```python
from build123d import *

# Parameters (mm, degrees)
SKETCH092_W             = 30.8
SKETCH092_H             = 12.5
PAD112_DEPTH            = 0.3
POCKET002_DEPTH         = 0.3
PAD113_DEPTH            = 5.5
POCKET003_DEPTH         = 5.5
FILLET014_R             = 0.75
SKETCH011_R             = 1.5
PAD114_DEPTH            = 5
BODY029_PLACEMENT_ANGLE = 180


with BuildPart() as part:
    # Sketch092 → Pad112 (new body)
    with BuildSketch(Plane(origin=(0, 3, 0), x_dir=(-1, 0, 0), z_dir=(0, 1, 0))):
        with Locations((0, 6.25)):
            Rectangle(SKETCH092_W, SKETCH092_H)
    extrude(amount=PAD112_DEPTH)

    # Sketch091 → Pocket002 (cut)
    with BuildSketch(Plane(origin=(0, 3, 0), x_dir=(-1, 0, 0), z_dir=(0, 1, 0))):
        with BuildLine():
            Line((-7, 10.175), (7, 10.175))
            ThreePointArc((7.391964, 9.675), (7.317662, 10.020388), (7, 10.175))
            Line((7.391964, 9.675), (5.67688, 2.69884))
            ThreePointArc((5.2, 2.325), (5.502973, 2.4296), (5.67688, 2.69884))
            Line((5.2, 2.325), (-5.2, 2.325))
            ThreePointArc((-5.67688, 2.69884), (-5.502973, 2.4296), (-5.2, 2.325))
            Line((-5.67688, 2.69884), (-7.391964, 9.675))
            ThreePointArc((-7, 10.175), (-7.317662, 10.020388), (-7.391964, 9.675))
        make_face()
    extrude(amount=POCKET002_DEPTH, mode=Mode.SUBTRACT)

    # Sketch091 → Pad113 (join)
    with BuildSketch(Plane(origin=(0, 3, 0), x_dir=(-1, 0, 0), z_dir=(0, 1, 0))):
        with BuildLine():
            Line((-7, 10.175), (7, 10.175))
            ThreePointArc((7.391964, 9.675), (7.317662, 10.020388), (7, 10.175))
            Line((7.391964, 9.675), (5.67688, 2.69884))
            ThreePointArc((5.2, 2.325), (5.502973, 2.4296), (5.67688, 2.69884))
            Line((5.2, 2.325), (-5.2, 2.325))
            ThreePointArc((-5.67688, 2.69884), (-5.502973, 2.4296), (-5.2, 2.325))
            Line((-5.67688, 2.69884), (-7.391964, 9.675))
            ThreePointArc((-7, 10.175), (-7.317662, 10.020388), (-7.391964, 9.675))
        make_face()
    extrude(amount=PAD113_DEPTH)

    # Sketch093 → Pocket003 (cut)
    with BuildSketch(Plane(origin=(0, 3, 0), x_dir=(-1, 0, 0), z_dir=(0, 1, 0))):
        with BuildLine():
            Line((-6, 9.18), (6, 9.18))
            ThreePointArc((6.390856, 8.68), (6.31732, 9.025285), (6, 9.18))
            Line((6.390856, 8.68), (5.098578, 3.485231))
            ThreePointArc((4.9, 3.33), (5.026026, 3.373413), (5.098578, 3.485231))
            Line((4.9, 3.33), (-4.9, 3.33))
            ThreePointArc((-5.098578, 3.485231), (-5.026026, 3.373413), (-4.9, 3.33))
            Line((-5.098578, 3.485231), (-6.390856, 8.68))
            ThreePointArc((-6, 9.18), (-6.31732, 9.025285), (-6.390856, 8.68))
        make_face()
    extrude(amount=POCKET003_DEPTH, mode=Mode.SUBTRACT)

    # Fillet014
    fillet014_edges = [part.edges().sort_by_distance(p)[0] for p in [
        (0, 8.5, 10.175),
        (7.317662, 8.5, 10.020388),
        (6.534422, 8.5, 6.18692),
        (5.502973, 8.5, 2.4296),
        (0, 8.5, 2.325),
        (-5.502973, 8.5, 2.4296),
        (-6.534422, 8.5, 6.18692),
        (-7.317662, 8.5, 10.020388),
    ]]
    fillet(fillet014_edges, radius=FILLET014_R)

    # Sketch011 → Pad114 (join)
    with BuildSketch(Plane(origin=(0, 3.3, 0), x_dir=(-1, 0, 0), z_dir=(0, 1, 0))):
        Polygon((-9.9, 4.893227), (-9.9, 7.606773), (-12.25, 8.963546), (-14.6, 7.606773), (-14.6, 4.893227), (-12.25, 3.536454), align=None)
        with Locations((-12.25, 6.25)):
            Circle(SKETCH011_R, mode=Mode.SUBTRACT)
        Polygon((14.6, 4.893227), (14.6, 7.606773), (12.25, 8.963546), (9.9, 7.606773), (9.9, 4.893227), (12.25, 3.536454), align=None)
        with Locations((12.25, 6.25)):
            Circle(SKETCH011_R, mode=Mode.SUBTRACT)
    extrude(amount=PAD114_DEPTH)


with BuildPart() as part_1:
    # Body029 placement: moved
    add(part.part.moved(Location((5.3, 0, 0))).rotate(Axis((5.3, 0, 0), (0, 0, 1)), BODY029_PLACEMENT_ANGLE))


solid = part_1.part
```
CAD build for the part. Positions are in the model's coordinates, mm. A direction names the side the tool comes from. Coordinates: 2 decimals unless noted, no trailing zeros. Order: outer loops, then holes, each group sorted by start corner. A loop starts at its lowest first (then second) coordinate and runs counter-clockwise, first axis right, second up. Notation, with made-up numbers: (-31.75, 35.25) - (18.25, 35.25) arc R22 cw to (18.25, 68.25) - close; hole circle Ø9 at (-33, 41). An arc over 180 degrees is marked (long way). Answer in a Markdown table with one row per item.
1. Pull direction Z, two halves, no side cores. Call faces 5 (the face through (11.054, -5.712, 6.119)), 6 (the face through (5, -5, 2.325)), 7 (the face through (16.4, -5.8, 8.3)): +Z half, -Z half, draft (parallel to the pull), parting line (faces both ways), or undercut.
Answer:
| item | result |
|---|---|
| face 5 | undercut |
| face 6 | -Z half |
| face 7 | +Z half |
2. 3-axis set-ups, long thin cutter, end or side, ignore diameter. For faces 1 (the face through (-8.1, -5.8, 8.3)), 2 (the face through (19.9, -6, 6)), 3 (the face through (-0.436, -5.712, 6.046)), 4 (the face through (18, -3.3, 6)): which of +Z, -Z, +X, -X, +Y, -Y reach the whole face in a straight line?
Answer:
| item | result |
|---|---|
| face 1 | +Z, -X, -Y |
| face 2 | +Z, -Z, +X, -Y |
| face 3 | +Y, -Y |
| face 4 | -Y |
3. Flat gauge pins, fed straight in: P1, Ø0.9, axis at x = -7, z = 6, coming from the -Y side; P2, Ø0.8, axis at y = -5.5, z = 6, coming from the +X side; P3, Ø2, axis at y = -6, z = 6, coming from the -X side; P4, Ø1, axis at x = 10, z = 9, coming from the -Y side. Where does each tip first touch, or does it go through?
Answer:
| item | result |
|---|---|
| P1 | y = -3.3 |
| P2 | x = 19.9 |
| P3 | x = -9.3 |
| P4 | y = -8.5 |
4. Slice it at B-B, the plane x = 6.5. List the corners of the cut face in (y, z) (3 decimals), then the cut area to 3 significant figures.
Answer:
| item | result |
|---|---|
| outline | (-8.5, 3.075) arc R0.75 ccw to (-7.75, 2.325) - (-3.3, 2.325) - (-3.3, 0) - (-3, 0) - (-3, 3.33) - (-8.5, 3.33) - close; (-8.5, 9.18) - (-3, 9.18) - (-3, 12.5) - (-3.3, 12.5) - (-3.3, 10.175) - (-7.75, 10.175) arc R0.75 ccw to (-8.5, 9.425) - close |
| area | 12.2 mm² |
5. Drill centre lines: L1, parallel to X at y = -7.15, z = 4; L2, parallel to Z at x = 5, y = -4.1 (3 decimals); L3, parallel to Y at x = 19.5, z = 10.25. Where is each one in solid material? Low to high. Write a range as from..to.
Answer:
| item | result |
|---|---|
| L1 | -7.75..-6.15, -0.7..0.07, 10.53..11.3, 16.75..18.35 |
| L2 | 2.325..3.33, 9.18..10.175 |
| L3 | -3.3..-3 |
6. Slice it at C-C, the plane x = 13. List the corners of the cut face in (y, z), then the cut area to 3 significant figures.
Answer:
| item | result |
|---|---|
| outline | (-3.3, 0) - (-3, 0) - (-3, 12.5) - (-3.3, 12.5) - close |
| area | 3.75 mm² |
7. Slice it at A-A, the plane y = -6.65. Give the number of separate pieces and of enclosed holes in the cut face, then the cut area to 3 significant figures.
Answer:
| item | result |
|---|---|
| separate pieces | 3 |
| enclosed holes | 3 |
| area | 59.2 mm² |
